Autodesk Inventor part; units mm, degrees
ref_plane "Work Plane1" through (9.305, 0, 0) normal (0, 0, 1) x (-1, 0, 0)
ref_plane "YZ Plane" through (0, 0, 0) normal (1, 0, 0) x (0, 1, 0)
ref_plane "XZ Plane" through (0, 0, 0) normal (0, 1, 0) x (-1, 0, 0)
sketch "Sketch1" plane through (0, 0, 0) normal (1, 0, 0) x (0, 1, 0)
  line L0 (1.5877, -2.75) -> (-1.5877, -2.75)
  line L1 (-1.5877, -2.75) -> (-3.1754, 0)
  line L2 (-3.1754, 0) -> (-1.5877, 2.75)
  line L3 (-1.5877, 2.75) -> (1.5877, 2.75)
  line L4 (1.5877, 2.75) -> (3.1754, 0)
  line L5 (3.1754, 0) -> (1.5877, -2.75)
  point P0 (0, 0)
  point P1 (0, 0)
  dimension "d0" = 6.3509
extrude "Body" add sketch "Sketch1" along normal blind 2.4
sketch "Sketch2" plane through (2.4, 0, 0) normal (1, 0, 0) x (0, 0, -1)
  circle A0 centre (0, 0) radius 2.3
  dimension "d7" = 4.6
extrude "Ring" add sketch "Sketch2" along normal blind 1.6
sketch "Sketch3" plane through (0, 0, 0) normal (0, 0, 1) x (1, 0, 0)
  line L0 (0, 1.5877) -> (0, 3.1754)
  line L1 (0, 3.1754) -> (2.4, 3.1754)
  line L2 (2.4, 1.5877) -> (2.4, 3.1754)
  line L3 (-0.48, 0) -> (2.88, 0)
  line L4 (0, 2.3) -> (0.5054, 3.1754)
  line L5 (1.8946, 3.1754) -> (2.4, 2.3)
  dimension "d3" = 30
  dimension "d4" = 30
  dimension "d5" = 4.6
  dimension "d6" = 4.6
revolve "Chamfer1" cut sketch "Sketch3" angle 360 about axis through (-10, 0, 0) along (1, 0, 0)
sketch "Sketch4" plane through (0, 0, 0) normal (-1, 0, 0) x (0, 0, 1)
  line L0 (0, -4.4456) -> (0, 4.4456)
  line L1 (-3.85, 0) -> (3.85, 0)
  point P0 (0, 0)
hole "Thread" at (0, 0, 0) direction (1, 0, 0) diameter 2.459 end through all
chamfer "Chamfer2" distance 0.2706 angle 30 1 edges at (0, 0, -1.2295) measured on face at (0, 1.9179, -0.2329)
chamfer "Chamfer3" distance 0.2706 angle 30 1 edges at (4, 0, -1.2295) measured on face at (4, -0.2816, -1.909)
ref_plane "Work Plane1" through (9.305, 0, 0) normal (0, 0, 1) x (-1, 0, 0)
equation "\"d0\" = 1.1547 * SW"
equation "\"d1\" = KOH1"
equation "\"d7\" = SD2"
equation "\"d8\" = KOH - KOH1"
equation "\"d3\" = ANG1"
equation "\"d4\" = ANG2"
equation "\"d5\" = SW0"
equation "\"d6\" = SW01"
equation "\"d10\" = -0.5 * GD1 + 0.5 * NND"
equation "\"d46\" = -0.5 * GD1 + 0.5 * NND"
equation "\"d12\" = -0.5 * GD1 + 0.5 * NND"
equation "\"d47\" = -0.5 * GD1 + 0.5 * NND"
equation "\"ANG1\" = 30deg"
equation "\"ANG2\" = 30deg"
equation "\"NND\" = 3"
equation "\"KOH1\" = 2.4"
equation "\"KOH\" = 4"
equation "\"SW\" = 5.5"
equation "\"SW0\" = 4.6"
equation "\"SW01\" = SW0"
equation "\"SD2\" = SW0"
equation "\"GUL\" = 0.541266 * PTC"
equation "\"THREADDIA\" = 3"
equation "\"TOA\" = 30deg"
equation "\"PTC\" = 0.5"
equation "\"GAL\" = 0.541266 * PTC"
equation "\"E0\" = 1.155 * SW"
properties part number "DIN 985 - M3" material "Steel, Mild"
Design review of the part built by this model. Coordinates are the model's own, in mm. Coordinates: 2 decimals unless noted, no trailing zeros. Write each loop counter-clockwise with the first axis right and the second up, starting at its lowest first coordinate (ties: lowest second). Pieces come first, ordered by that corner, then holes.
1) Mouldability with a two-part tool opening along Z and no side actions: class faces 1 (the cylindrical face through (2.026, 0.748, -0.976)), 2 (the cylindrical face through (3.189, 1.4, 1.825)), 3 (the flat face through (1.187, -2.37, -1.394)), 4 (the flat face through (4, -2, 0)) as +Z half, -Z half, draft (parallel to the pull), parting line (faces both ways), or undercut.
2) Add section A-A (y = 0). Write out the cut boundary in (x, z).
3) To check wall thickness, follow L1, parallel to Z at x = 1.25, y = 0; L2, parallel to Z at x = 3.05, y = 0; L3, parallel to Y at x = 3, z = -0.5 (3 decimals). State the ranges of each line that lie inside material, in increasing order.
4) Add section B-B (x = 1). Write out the cut boundary in (y, z), plus the area to 3 significant figures.
5) Insertion check: pin 1 (2 mm diameter, centred on x = 3, y = -2, fed in from +Z); pin 2 (2 mm diameter, centred on x = 2, z = -2, fed in from -Y); pin 3 (1.5 mm diameter, centred on x = 3.5, z = -2, fed in from +Y). Each pin has a flat end and moves straight along its axis. Give the tip position at first contact, or say it passes through.
6) Add section C-C (x = 2.85). Write out the cut boundary in (y, z), plus the area to 3 significant figures.
Check result:
1. face 1: undercut
1. face 2: parting line
1. face 3: -Z half
1. face 4: draft
2. outline: (0, -2.3) - (0.26, -2.75) - (2.14, -2.75) - (2.4, -2.3) - (4, -2.3) - (4, -1.5) - (3.84, -1.23) - (0.16, -1.23) - (0, -1.5) - close; (0, 1.5) - (0.16, 1.23) - (3.84, 1.23) - (4, 1.5) - (4, 2.3) - (2.4, 2.3) - (2.14, 2.75) - (0.26, 2.75) - (0, 2.3) - close
3. L1: z = -2.75 to -1.23, 1.23 to 2.75
3. L2: z = -2.3 to -1.23, 1.23 to 2.3
3. L3: y = -2.245 to -1.123, 1.123 to 2.245
4. outline: (-3.18, 0) - (-1.59, -2.75) - (1.59, -2.75) - (3.18, 0) - (1.59, 2.75) - (-1.59, 2.75) - close; hole circle Ø2.46 at (0, 0)
4. area: 21.4 mm2
5. pin 1: stops at z = 2.37
5. pin 2: stops at y = -2.6
5. pin 3: stops at y = 1.93
6. outline: circle Ø4.6 at (0, 0); hole circle Ø2.46 at (0, 0)
6. area: 11.9 mm2
